Input: part model. Units: mm. Frame: model coordinates. Face numbers are marked on the shaded views. A direction names the side the tool comes from. Round coordinates to 2 decimals unless told otherwise and drop trailing zeros. Loops run counter-clockwise (first coordinate to the right, second up) from the corner with the lowest first, then second, coordinate; pieces in that order, holes last. Notation, with made-up numbers: (-32.5, 58) -> (20.5, 58) arc R22 ccw to (20.5, 85) -> close; hole circle Ø2 at (84.5, -15). An arc over 180 degrees is marked (long way). One line per question, with ' | ' between items. Start each with the question number.
Q1. Cut plane C-C on y = -6. Return loops of the section in (x, z).
Q2. Access query for the marked faces 1, 2 and 3. Directions: +Z, -Z, +X, -X, +Y, -Y. A direction counts if a zero-diameter tool reaches every point of the face in a straight line with its end or side. Return the directions, or none.
Q3. Cut plane A-A on x = 0. Return loops of the section in (y, z), and give its area (3 significant figures).
Q4. Material intervals for L1, parallel to Y at x = 0, z = 1.6; L2, parallel to Y at x = 0.5, z = 1.4; L3, parallel to Y at x = 0, z = 3.95, sorted ascending.
Q5. Contact query for flat-ended pins moving along their axis: P1, Ø2, axis at y = -4.5, z = 1, coming from the -X side; P2, Ø3, axis at x = -0.5, y = -0.5, coming from the -Z side; P3, Ø1.3, axis at x = 0, y = 6, coming from the +Z side; P4, Ø4, axis at x = -6, y = -2, coming from the +Z side. Output: stop coordinate, or through.
Q6. Cut plane D-D on z = 1.5. State how many separate pieces and enclosed holes the cut face has, and give its area (3 significant figures).
from build123d import *

# Parameters (mm, degrees)
F0_R     = 4.5
F0_R_2   = 3
F1_DEPTH = 1.2
F2_R     = 8
F2_R_2   = 0.8
F2_R_3   = 4.5
F2_R_4   = 3
F3_DEPTH = 2
F4_R     = 4
F4_R_2   = 1.55
F5_DEPTH = 1


with BuildPart() as f1:
    # F0 (on Top) → F1 (new body)
    with BuildSketch(Plane.XY):
        Circle(F0_R)
        Circle(F0_R_2, mode=Mode.SUBTRACT)
    extrude(amount=F1_DEPTH)

    # F2 (on face) → F3 (join)
    with BuildSketch(Plane.XY.offset(1.2)):
        Circle(F2_R)
        with Locations((-4.2426406871, -4.2426406871)):
            Circle(F2_R_2, mode=Mode.SUBTRACT)
        with Locations((0, -6)):
            Circle(F2_R_2, mode=Mode.SUBTRACT)
        with Locations((4.2426406871, -4.2426406871)):
            Circle(F2_R_2, mode=Mode.SUBTRACT)
        with Locations((-6, 0)):
            Circle(F2_R_2, mode=Mode.SUBTRACT)
        with Locations((-4.2426406871, 4.2426406871)):
            Circle(F2_R_2, mode=Mode.SUBTRACT)
        Circle(F2_R_3, mode=Mode.SUBTRACT)
        with Locations((6, 0)):
            Circle(F2_R_2, mode=Mode.SUBTRACT)
        with Locations((0, 6)):
            Circle(F2_R_2, mode=Mode.SUBTRACT)
        with Locations((4.2426406871, 4.2426406871)):
            Circle(F2_R_2, mode=Mode.SUBTRACT)
        Circle(F2_R_3)
        Circle(F2_R_4, mode=Mode.SUBTRACT)
    extrude(amount=F3_DEPTH)

    # F4 (on face) → F5 (join)
    with BuildSketch(Plane.XY.offset(3.2)):
        Circle(F4_R)
        Circle(F4_R_2, mode=Mode.SUBTRACT)
    extrude(amount=F5_DEPTH)


solid = f1.part
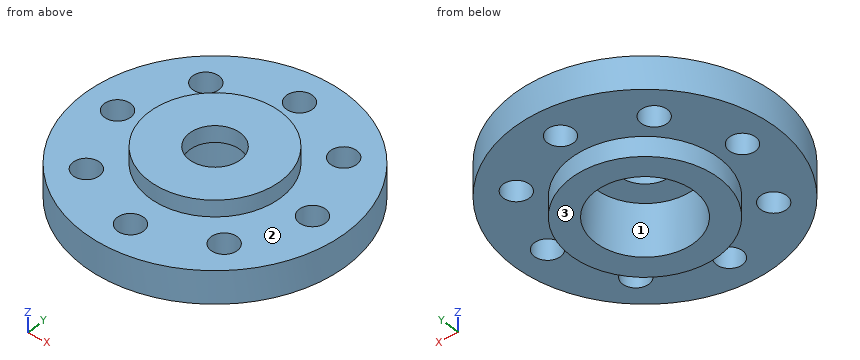
Results:
1) outline: (-5.29, 1.2) -> (-0.8, 1.2) -> (-0.8, 3.2) -> (-5.29, 3.2) -> close; (0.8, 1.2) -> (5.29, 1.2) -> (5.29, 3.2) -> (0.8, 3.2) -> close
2) face 1: -Z | face 2: +Z | face 3: -Z, +X, -X, +Y, -Y
3) outline: (-8, 1.2) -> (-6.8, 1.2) -> (-6.8, 3.2) -> (-8, 3.2) -> close; (-5.2, 1.2) -> (-4.5, 1.2) -> (-4.5, 0) -> (-3, 0) -> (-3, 3.2) -> (-1.55, 3.2) -> (-1.55, 4.2) -> (-4, 4.2) -> (-4, 3.2) -> (-5.2, 3.2) -> close; (1.55, 3.2) -> (3, 3.2) -> (3, 0) -> (4.5, 0) -> (4.5, 1.2) -> (5.2, 1.2) -> (5.2, 3.2) -> (4, 3.2) -> (4, 4.2) -> (1.55, 4.2) -> close; (6.8, 1.2) -> (8, 1.2) -> (8, 3.2) -> (6.8, 3.2) -> close | area: 22.1 mm^2
4) L1: -8 to -6.8, -5.2 to -3, 3 to 5.2, 6.8 to 8 | L2: -7.98 to -6.62, -5.38 to -2.96, 2.96 to 5.38, 6.62 to 7.98 | L3: -4 to -1.55, 1.55 to 4
5) P1: x = -7.18 | P2: z = 3.2 | P3: through | P4: z = 3.2
6) separate pieces: 1 | enclosed holes: 9 | area: 157 mm^2
